Autodesk Inventor part; units mm, degrees
ref_plane "YZ Plane" through (0, 0, 0) normal (1, 0, 0) x (0, 1, 0)
ref_plane "XZ Plane" through (0, 0, 0) normal (0, 1, 0) x (-1, 0, 0)
ref_plane "XY Plane" through (0, 0, 0) normal (0, 0, 1) x (1, 0, 0)
sketch "Sketch4" plane through (0, 0, 0) normal (0, 1, 0) x (-1, 0, 0)
  circle A0 centre (0, 0) radius 1.5
extrude "Extrusion2" add sketch "Sketch4" along normal mid plane 139.5
sketch "Sketch13" plane through (0, 0, 0) normal (1, 0, 0) x (0, 1, 0)
  line L0 (70.3754, -0.5) -> (63.75, -0.5)
  line L1 (63.75, -0.5) -> (63.75, -2.4686)
  line L2 (63.75, -2.4686) -> (70.3754, -2.4686)
  line L3 (70.3754, -2.4686) -> (70.3754, -0.5)
  line L4 (-69.75, -1.5) -> (69.75, -1.5)
  line L5 (69.75, -1.5) -> (69.75, 1.5)
  line L6 (-0.35, 2.5026) -> (-30.35, 2.5026)
  line L7 (-30.35, 2.5026) -> (-30.35, 0.5)
  line L8 (-30.35, 0.5) -> (-0.35, 0.5)
  line L9 (-0.35, 0.5) -> (-0.35, 2.5026)
  line L10 (-69.75, 1.5) -> (69.75, 1.5)
  line L11 (-69.75, 1.5) -> (-69.75, -1.5)
  point P0 (0, 0)
  point P1 (-0.35, 1.5)
  point P2 (-30.35, 1.5)
  point P3 (69.75, -0.5)
  point P4 (63.75, -1.5)
  dimension "d89" = 1
  dimension "d90" = 6
  dimension "d91" = 1
  dimension "d92" = 30
  dimension "d93" = 39.4
extrude "Extrusion9" cut sketch "Sketch13" against normal through all both and the other way through all contours L5 L4 L1 L0 | L9 L8 L7 L10
properties part number "Wheel Shaft 125mm" material "Bronze, Soft Tin"
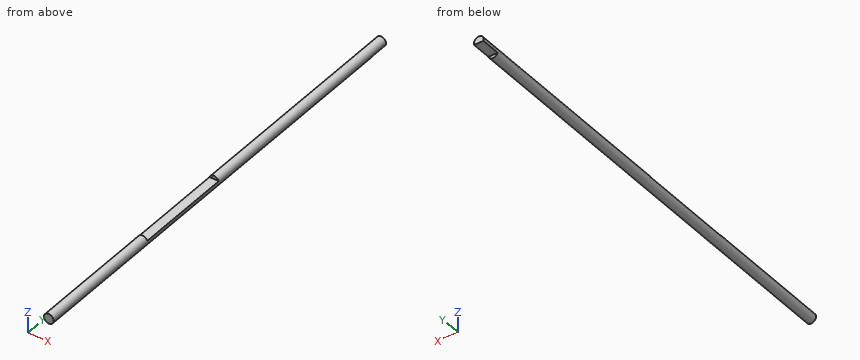
Can you work these out from the model? Positions are in its coordinate system, mm. Give positions to 0.01 mm unless a question says otherwise; leave off trailing zeros. Loops run counter-clockwise (first coordinate to the right, second up) from the corner with the lowest first, then second, coordinate; pieces in that order, holes last. Notation, with made-up numbers: (-3.75, -27) -> (48.25, -27) arc R10 cw to (48.25, -17) -> close; hole circle Ø1 at (15, 38). An arc over 180 degrees is marked (long way). Use one line per item in the form item = value.
1) I need wall thicknesses on line 1 along Y through (x, z) = (-0.4, 0.95); line 2 along X through (y, z) = (43.5, -0.25); line 3 along Y through (x, z) = (0, -0.6). Which ranges of each line are inside material? Lowest first, please.
Answers:
line_1 = -69.75 to -30.35, -0.35 to 69.75
line_2 = -1.48 to 1.48
line_3 = -69.75 to 63.75
2) Will these pins go through, and if not, where does the flat tip stop? pin 1 (0.5 mm diameter, centred on x = -0.5, z = -1, fed in from +Y); pin 2 (0.8 mm diameter, centred on x = 0.5, y = -13.5, fed in from +Z); pin 3 (0.8 mm diameter, centred on x = 0, y = 66.5, fed in from -Z); pin 4 (1 mm diameter, centred on x = 0.5, y = -55.5, fed in from +Z).
Answers:
pin_1 = 63.75
pin_2 = 0.5
pin_3 = -0.5
pin_4 = 1.5
3) If we section it at B-B (y = -44): Please give me the cut outline in (x, z).
Answers:
outline = circle Ø3 at (0, 0)
4) If we section it at A-A (x = 0): Please give me the cut outline in (y, z), plus the area to 4 significant figures.
Answers:
outline = (-69.75, -1.5) -> (63.75, -1.5) -> (63.75, -0.5) -> (69.75, -0.5) -> (69.75, 1.5) -> (-0.35, 1.5) -> (-0.35, 0.5) -> (-30.35, 0.5) -> (-30.35, 1.5) -> (-69.75, 1.5) -> close
area = 382.5 mm²
